Geometry check sheet. Reference: the model listing, model coordinates, mm. Face numbers are marked on the shaded views. A direction names the side the tool comes from. Give positions to 0.01 mm unless a question says otherwise; leave off trailing zeros. Loops run counter-clockwise (first coordinate to the right, second up) from the corner with the lowest first, then second, coordinate; pieces in that order, holes last.
1. Cross-section at D-D, the plane z = 3. Record the cut outline in (x, y), plus the area to 3 significant figures.
2. Cross-section at C-C, the plane z = 26.25. State how many separate pieces and enclosed holes the cut face has, plus the area to 3 significant figures.
3. Go/stop test with flat-tipped pins: pin 1 Ø1 at (y, z) = (-19, 22) entering from -X; pin 2 Ø9 at (x, y) = (-24.67, -24.67) entering from -Z; pin 3 Ø2 at (y, z) = (23, 26) entering from -X; pin 4 Ø17.5 at (x, y) = (13.5, -18.5) entering from +Z. Record where each tip stops, or that it passes through.
4. Cross-section at A-A, the plane y = 0. Record the cut outline in (x, z).
5. Material ranges on L1, parallel to Y at x = -0.5, z = 3.75; L2, parallel to X at y = 0, z = 21.75; L3, parallel to Z at x = 28.5, y = -18, recorded low to high.
6. Tool access check on the marked faces 4, 5 and 6. Record the directions out of +Z, -Z, +X, -X, +Y, -Y that give a thin tool (end or side, any length) a straight path to the whole face; none if there is none.
7. Cross-section at B-B, the plane x = 35. Record the cut outline in (y, z).
8. Release check for a two-part mould opening along Y. For the marked faces 1, 2 and 3 record: +Y half, -Y half, draft (parallel to the pull), parting line (faces both ways), or undercut.
from build123d import *

# Parameters (mm, degrees)
F0_R      = 41.5
F1_DEPTH  = 29
F2_R      = 41.5
F2_R_2    = 16.5
F3_DEPTH  = 11.5
F4_R      = 11
F5_DEPTH  = 29.001
F6_R      = 12.75
F7_DEPTH  = 5
F8_R      = 1.5
F9_DEPTH  = 29.001
F10_D     = 7
F11_W     = 2
F11_H     = 1.4
F13_D     = 2.5
F15_DEPTH = 9
F16_R     = 6
F17_DEPTH = 13


with BuildPart() as f1:
    # F0 (on Top) → F1 (new body)
    with BuildSketch(Plane.XY):
        Circle(F0_R)
    extrude(amount=F1_DEPTH)

    # F2 (on face) → F3 (cut)
    with BuildSketch(Plane(origin=(0, 0, 0), x_dir=(1, 0, 0), z_dir=(0, 0, -1))):
        Circle(F2_R)
        Circle(F2_R_2, mode=Mode.SUBTRACT)
    extrude(amount=-F3_DEPTH, mode=Mode.SUBTRACT)

    # F4 (on face) → F5 (cut, through all)
    with BuildSketch(Plane(origin=(0, 0, 0), x_dir=(1, 0, 0), z_dir=(0, 0, -1))):
        Circle(F4_R)
    extrude(amount=-F5_DEPTH, mode=Mode.SUBTRACT)

    # F6 (on face) → F7 (cut)
    with BuildSketch(Plane(origin=(0, 0, 0), x_dir=(1, 0, 0), z_dir=(0, 0, -1))):
        Circle(F6_R)
    extrude(amount=-F7_DEPTH, mode=Mode.SUBTRACT)

    # F8 (on face) → F9 (cut, through all)
    with BuildSketch(Plane.XY.offset(29)):
        with Locations((-9.203227, 33.048392)):
            Circle(F8_R)
        with Locations((-0.27397, -34.776049)):
            Circle(F8_R)
    extrude(amount=-F9_DEPTH, mode=Mode.SUBTRACT)

    # F10 (through all)
    with Locations(Plane.XY.offset(29)):
        with Locations((-0.27397, 34.223951), (33.050471, -9.205307), (-24.669154, -24.671233)):
            Hole(F10_D / 2)

    # F11 (on Front) → F12 (revolve, cut)
    with BuildSketch(Plane.XZ):
        with Locations((29.24357, 28.3)):
            Rectangle(F11_W, F11_H)
    revolve(axis=Axis((0, 0, 11.697991), (0, 0, 1)), mode=Mode.SUBTRACT)

    # F13 (through all)
    with Locations(Plane.XY.offset(29)):
        with Locations((-0.27397, 26.223951)):
            Hole(F13_D / 2)

    # F14 (on face) → F15 (cut)
    with BuildSketch(Plane.XY.offset(29)):
        with BuildLine():
            Line((16.103088, -22.212727), (24.192653, -13.349379))
            ThreePointArc((24.192653, -13.349379), (23.621079, -7.823223), (18.07709, -8.182768))
            Line((18.07709, -8.182768), (9.987525, -17.046116))
            ThreePointArc((9.987525, -17.046116), (10.361111, -22.806624), (16.103088, -22.212727))
        make_face()
    extrude(amount=-F15_DEPTH, mode=Mode.SUBTRACT)

    # F16 (on face) → F17 (cut)
    with BuildSketch(Plane(origin=(0, 0, 11.5), x_dir=(1, 0, 0), z_dir=(0, 0, -1))):
        with Locations((21.92031, 21.92031)):
            Circle(F16_R)
    extrude(amount=-F17_DEPTH, mode=Mode.SUBTRACT)


solid = f1.part
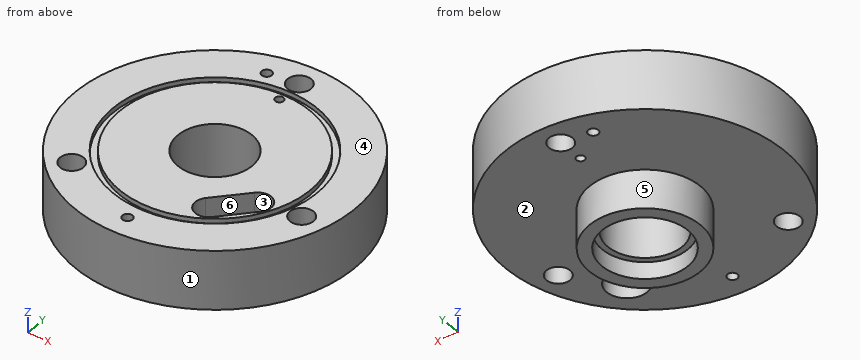
Result:
1. outline: circle Ø33 at (0, 0); hole circle Ø25.5 at (0, 0)
1. area: 345 mm2
2. separate pieces: 1
2. enclosed holes: 8
2. area: 4,750 mm2
3. pin 1: stops at x = -37.15
3. pin 2: stops at z = 11.5
3. pin 3: stops at x = -35.19
3. pin 4: stops at z = 29
4. outline: (-41.5, 11.5) - (-16.5, 11.5) - (-16.5, 0) - (-12.75, 0) - (-12.75, 5) - (-11, 5) - (-11, 29) - (-28.24, 29) - (-28.24, 27.6) - (-30.24, 27.6) - (-30.24, 29) - (-41.5, 29) - close; (11, 5) - (12.75, 5) - (12.75, 0) - (16.5, 0) - (16.5, 11.5) - (41.5, 11.5) - (41.5, 29) - (30.24, 29) - (30.24, 27.6) - (28.24, 27.6) - (28.24, 29) - (11, 29) - close
5. L1: y = -16.49 to -12.74, 12.74 to 16.49
5. L2: x = -41.5 to -11, 11 to 41.5
5. L3: z = 11.5 to 29
6. face 4: +Z, +X, -X, +Y, -Y
6. face 5: -Z
6. face 6: +Z
7. outline: (-22.3, 11.5) - (-12.11, 11.5) - (-12.11, 29) - (-22.3, 29) - close; (-6.3, 11.5) - (22.3, 11.5) - (22.3, 29) - (-6.3, 29) - close
8. face 1: parting line
8. face 2: draft
8. face 3: undercut
